Autodesk Fusion 360 part; units mm, degrees
sketch "Skizze1" plane through (0, 0, 0) normal (0, 0, 1) x (1, 0, 0)
  line L0 (0, 0) -> (40, 0)
  line L1 (40, 0) -> (40, 110)
  line L2 (40, 110) -> (0, 110)
  line L3 (0, 110) -> (0, 0)
  dimension "d1" = 40
  dimension "d2" = 110
extrude "Extrusion1" add sketch "Skizze1" along normal blind 9
sketch "Skizze2" plane through (0, 0, 9) normal (0, 0, 1) x (-1, 0, 0)
  line L0 (0, -110) -> (0, 0)
  line L1 (0, 0) -> (-40, 0)
  line L2 (-40, 0) -> (-40, -110)
  line L3 (-40, -110) -> (0, -110)
  line L4 (-40, 0) -> (-35, 0)
  line L5 (-35, 0) -> (-35, -6)
  line L6 (-35, -6) -> (-40, -6)
  line L7 (-40, -6) -> (-40, 0)
  line L8 (0, 0) -> (-6, 0)
  line L9 (-6, 0) -> (-6, -6)
  line L10 (-6, -6) -> (0, -6)
  line L11 (0, -6) -> (0, 0)
  line L12 (0, -110) -> (-6, -110)
  line L13 (-6, -110) -> (-6, -104)
  line L14 (-6, -104) -> (0, -104)
  line L15 (0, -104) -> (0, -110)
  line L16 (-40, -110) -> (-34, -110)
  line L17 (-34, -110) -> (-34, -104)
  line L18 (-34, -104) -> (-40, -104)
  line L19 (-40, -104) -> (-40, -110)
  line L20 (-40, 0) -> (-34, 0)
  line L21 (-34, 0) -> (-34, -6)
  line L22 (-34, -6) -> (-40, -6)
  line L23 (-40, -6) -> (-40, 0)
  line L24 (-40, -110) -> (0, -110)
  line L25 (0, -110) -> (0, -71)
  line L26 (0, -71) -> (-40, -71)
  line L27 (-40, -71) -> (-40, -110)
  line L28 (0, 0) -> (-40, 0)
  line L29 (-40, 0) -> (-40, -39)
  line L30 (-40, -39) -> (0, -39)
  line L31 (0, -39) -> (0, 0)
  line L32 (-40, -39) -> (-34, -39)
  line L33 (-34, -39) -> (-34, -33)
  line L34 (-34, -33) -> (-40, -33)
  line L35 (-40, -33) -> (-40, -39)
  line L36 (0, -39) -> (-6, -39)
  line L37 (-6, -39) -> (-6, -33)
  line L38 (-6, -33) -> (0, -33)
  line L39 (0, -33) -> (0, -39)
  line L40 (0, -71) -> (-6, -71)
  line L41 (-6, -71) -> (-6, -77)
  line L42 (-6, -77) -> (0, -77)
  line L43 (0, -77) -> (0, -71)
  line L44 (-40, -71) -> (-34, -71)
  line L45 (-34, -71) -> (-34, -77)
  line L46 (-34, -77) -> (-40, -77)
  line L47 (-40, -77) -> (-40, -71)
  circle A0 centre (-6, -6) radius 2.75
  circle A1 centre (-34, -6) radius 2.75
  circle A2 centre (-6, -33) radius 2.75
  circle A3 centre (-34, -33) radius 2.75
  circle A4 centre (-34, -77) radius 2.75
  circle A5 centre (-6, -77) radius 2.75
  circle A6 centre (-6, -104) radius 2.75
  circle A7 centre (-34, -104) radius 2.75
  dimension "d5" = 6
  dimension "d6" = 6
  dimension "d7" = 6
  dimension "d8" = 6
  dimension "d9" = 6
  dimension "d10" = 6
  dimension "d11" = 6
  dimension "d12" = 6
  dimension "d13" = 6
  dimension "d14" = 40
  dimension "d15" = 39
  dimension "d16" = 40
  dimension "d17" = 39
  dimension "d18" = 6
  dimension "d19" = 6
  dimension "d20" = 6
  dimension "d21" = 6
  dimension "d22" = 6
  dimension "d23" = 6
  dimension "d24" = 6
  dimension "d25" = 6
  dimension "d26" = 5.5
  dimension "d27" = 5.5
  dimension "d28" = 5.5
  dimension "d29" = 5.5
  dimension "d30" = 5.5
  dimension "d31" = 5.5
  dimension "d32" = 5.5
  dimension "d33" = 5.5
extrude "Extrusion2" cut sketch "Skizze2" against normal blind 10 contours L13 L14 A6 | L13 L14 A6 | L41 L42 A5 | L41 L42 A5 | L17 L18 A7 | L17 L18 A7 | L37 L38 A2 | L37 L38 A2 | L45 L46 A4 | L45 L46 A4 | L9 L10 A0 | L9 L10 A0 | L33 L34 A3 | L33 L34 A3 | L6 L21 L22 A1 | L5 L21 L22 A1 | L5 L6 L22 A1
extrude "Extrusion11" cut 1 faces at (24.2083, 48.4605, 9) along direction (0, 0, -1) blind 1
sketch "Skizze10" plane through (0, 0, 0) normal (0, 0, 1) x (1, 0, 0)
  line L0 (0, 0) -> (0, 110)
  line L1 (0, 55) -> (0, 40)
  line L2 (0, 40) -> (-30, 40)
  line L3 (-30, 70) -> (0, 70)
  line L4 (0, 70) -> (0, 40)
  line L5 (-30, 70) -> (0, 70)
  line L6 (0, 70) -> (0, 77)
  line L7 (0, 77) -> (-30, 77)
  line L8 (-30, 77) -> (-30, 70)
  line L9 (-30, 40) -> (0, 40)
  line L10 (0, 40) -> (0, 33)
  line L11 (0, 33) -> (-30, 33)
  line L12 (-30, 33) -> (-30, 40)
  line L13 (0, 77) -> (-5, 77)
  line L14 (-5, 77) -> (-5, 110)
  line L15 (-5, 110) -> (0, 110)
  line L16 (0, 110) -> (0, 77)
  line L17 (0, 33) -> (-5, 33)
  line L18 (-5, 33) -> (-5, 0)
  line L19 (-5, 0) -> (0, 0)
  line L20 (0, 0) -> (0, 33)
  dimension "d69" = 15
  dimension "d70" = 30
  dimension "d71" = 30
  dimension "d72" = 7
  dimension "d73" = 7
extrude "Extrusion12" add sketch "Skizze10" along normal blind 38
sketch "Skizze11" plane through (0, 0, 0) normal (0, 0, 1) x (1, 0, 0)
  line L0 (-5, 0) -> (-5, 33)
  line L1 (-5, 33) -> (-30, 33)
  line L2 (-30, 33) -> (-5, 0)
  line L3 (-5, 110) -> (-5, 77)
  line L4 (-5, 77) -> (-30, 77)
  line L5 (-5, 110) -> (-30, 77)
extrude "Extrusion13" add sketch "Skizze11" along normal blind 5
extrude "Extrusion14" add 2 faces at (-13.3333, 88, 5) (-13.3333, 22, 5) along direction (0, 0, 1) blind 5 from surface at 28
sketch "Skizze12" plane through (0, 33, 0) normal (0, -1, 0) x (1, 0, 0)
  line L0 (-5, 33) -> (-30, 33)
  line L1 (-30, 33) -> (-30, 5)
  line L2 (-30, 5) -> (-5, 5)
  line L3 (-5, 5) -> (-5, 33)
  line L4 (-30, 33) -> (-15, 33)
  line L5 (-15, 33) -> (-15, 5)
  line L6 (-15, 33) -> (-15, 26)
  line L7 (-15, 5) -> (-15, 12)
  circle A0 centre (-15, 12) radius 3.5
  circle A1 centre (-15, 26) radius 3.5
  dimension "d81" = 15
  dimension "d82" = 7
  dimension "d83" = 7
  dimension "d84" = 7
  dimension "d85" = 7
extrude "Extrusion15" cut sketch "Skizze12" against normal blind 95 contours L5 L6 A1 | L5 L6 A1 | L5 L7 A0 | L5 L7 A0
Design review of the part built by this model. Coordinates are the model's own, in mm. A direction names the side the tool comes from. Give positions to 0.01 mm unless a question says otherwise; leave off trailing zeros. Order: outer loops, then holes, each group sorted by start corner. A loop starts at its lowest first (then second) coordinate and runs counter-clockwise, first axis right, second up.
1. For pin 1 Ø7 at (x, y) = (34, 6) entering from +Z; pin 2 Ø12 at (y, z) = (89.5, 20) entering from +X; pin 3 Ø1.5 at (x, z) = (-20.5, 16.5) entering from +Y, all flat-tipped, find the tip position at first contact; note any pin that passes through.
Solution:
pin 1: stops at z = 8
pin 2: stops at x = 0
pin 3: stops at y = 77
2. Add section B-B, the plane x = 6. State the section outline as (y, z) points.
Solution:
outline: (0, 0) - (3.25, 0) - (3.25, 8) - (0, 8) - close; (8.75, 0) - (30.25, 0) - (30.25, 8) - (8.75, 8) - close; (35.75, 0) - (74.25, 0) - (74.25, 8) - (35.75, 8) - close; (79.75, 0) - (101.25, 0) - (101.25, 8) - (79.75, 8) - close; (106.75, 0) - (110, 0) - (110, 8) - (106.75, 8) - close
3. Mouldability with a two-part tool opening along Y and no side actions: class faces 1 (the cylindrical face through (4.52, 74.68, 4.06)), 2 (the flat face through (12.4, 0, 7.7)), 3 (the flat face through (-12, 86, 33)) as +Y half, -Y half, draft (parallel to the pull), parting line (faces both ways), or undercut.
Solution:
face 1: undercut
face 2: -Y half
face 3: draft
4. To check wall thickness, follow L1, parallel to X at y = 33, z = 3.25; L2, parallel to X at y = 104, z = 5.75; L3, parallel to Y at x = 6, z = 2.5. State the ranges of each line that lie inside material, in increasing order.
Solution:
L1: x = -30 to 3.25, 8.75 to 31.25, 36.75 to 40
L2: x = -5 to 3.25, 8.75 to 31.25, 36.75 to 40
L3: y = 0 to 3.25, 8.75 to 30.25, 35.75 to 74.25, 79.75 to 101.25, 106.75 to 110
5. Add section A-A, the plane z = 12. State the section outline as (x, y) points.
Solution:
outline: (-30, 33) - (-18.5, 33) - (-18.5, 40) - (-30, 40) - close; (-30, 70) - (-18.5, 70) - (-18.5, 77) - (-30, 77) - close; (-11.5, 33) - (-5, 33) - (-5, 0) - (0, 0) - (0, 40) - (-11.5, 40) - close; (-11.5, 70) - (0, 70) - (0, 110) - (-5, 110) - (-5, 77) - (-11.5, 77) - close
6. Tool access review of faces 4 (the flat face through (0, 55, 4)), 5 (the flat face through (-12, 86, 5)), 6 (the flat face through (0, 20, 23)), 7 (the flat face through (-5, 17, 19)): name each direction out of +Z, -Z, +X, -X, +Y, -Y from which nothing blocks a thin tool from reaching the whole face with its end or side.
Solution:
face 4: +Z, -Z, -X
face 5: -X, +Y
face 6: +Z, +X, +Y, -Y
face 7: -X, -Y
7. Add section C-C, the plane z = 20. State the section outline as (x, y) points, then the cut area to 3 significant figures.
Solution:
outline: (-30, 33) - (-5, 33) - (-5, 0) - (0, 0) - (0, 40) - (-30, 40) - close; (-30, 70) - (0, 70) - (0, 110) - (-5, 110) - (-5, 77) - (-30, 77) - close
area: 750 mm2
8. Add section D-D, the plane y = 37.5. State the section outline as (x, z) points, then the cut area to 3 significant figures.
Solution:
outline: (-30, 0) - (40, 0) - (40, 8) - (0, 8) - (0, 38) - (-30, 38) - close; hole circle Ø7 at (-15, 12); hole circle Ø7 at (-15, 26)
area: 1,380 mm2
